from build123d import *

# Parameters (mm, degrees)
BOSS_EXTRUDE1_DEPTH = 3.175
SKETCH2_R           = 2.25
CUT_EXTRUDE1_DEPTH  = 126.120784145
FILLET1_R           = 2.54


with BuildPart() as part:
    # Sketch1 → Boss-Extrude1 (new body)
    with BuildSketch(Plane.XY):
        with BuildLine():
            Line((0, 25.4), (0, 0))
            Line((0, 0), (114.3, 0))
            Line((114.3, 0), (114.3, 50.8))
            Line((114.3, 50.8), (25.4, 50.8))
            ThreePointArc((25.4, 50.8), (17.960512242, 32.839487758), (0, 25.4))
        make_face()
    extrude(amount=BOSS_EXTRUDE1_DEPTH)

    # Sketch2 → Cut-Extrude1 (cut, through all)
    with BuildSketch(Plane.XY.offset(3.175)):
        with BuildLine():
            Line((114.3, 50.8), (69.85, 50.8))
            ThreePointArc((69.85, 50.8), (101.175009976, 37.886844698), (114.3, 6.65))
            Line((114.3, 6.65), (114.3, 50.8))
        make_face()
        with Locations((85.725, 6.65)):
            Circle(SKETCH2_R)
        with BuildLine():
            Line((90.17, 28.843472461), (33.02, 28.843472461))
            ThreePointArc((33.02, 28.843472461), (29.845, 25.668472461), (33.02, 22.493472461))
            Line((33.02, 22.493472461), (90.17, 22.493472461))
            ThreePointArc((90.17, 22.493472461), (93.345, 25.668472461), (90.17, 28.843472461))
        make_face()
        with Locations((28.575, 6.65)):
            Circle(SKETCH2_R)
    extrude(amount=-CUT_EXTRUDE1_DEPTH, mode=Mode.SUBTRACT)

    # Fillet1
    fillet1_edges = [part.edges().sort_by_distance(p)[0] for p in [
        (114.3, 0, 1.5875),
        (0, 0, 1.5875),
        (0, 25.4, 1.5875),
        (25.4, 50.8, 1.5875),
    ]]
    fillet(fillet1_edges, radius=FILLET1_R)


solid = part.part
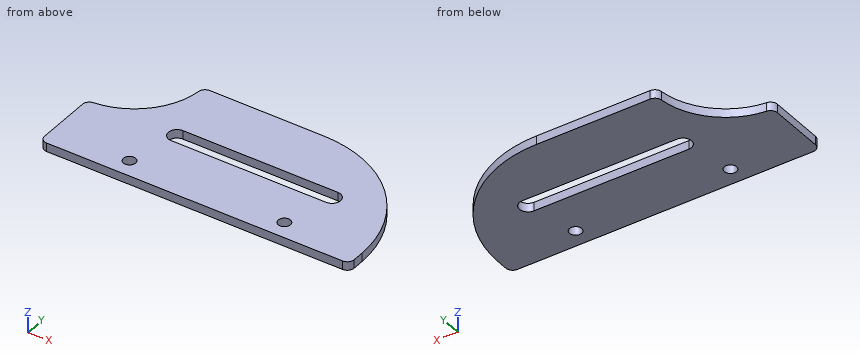
Build history of the part. All positions in model axes, mm. Round coordinates to 2 decimals unless told otherwise and drop trailing zeros. Write each loop counter-clockwise with the first axis right and the second up, starting at its lowest first coordinate (ties: lowest second). Pieces come first, ordered by that corner, then holes. Notation, with made-up numbers: (-19, -16) - (-5, -16) arc R33 cw to (-5, 13) - close; hole circle Ø10 at (70.5, 83). An arc over 180 degrees is marked (long way). Use CSV: the item, a comma, the result in double quotes.
(1) Band-saw the part on C-C (y = 27). Write the cut outline in (x, z) (3 decimals), plus the area to 3 significant figures.
Response:
outline,"(8.872, 0) - (30.138, 0) - (30.138, 3.175) - (8.872, 3.175) - close; (93.052, 0) - (109.213, 0) - (109.213, 3.175) - (93.052, 3.175) - close"
area,"119 mm²"
(2) Pin check, flat tips, straight feed: P1, Ø4, axis at x = 28.575, y = 6.65, coming from the +Z side; P2, Ø1, axis at y = 23, z = 2.5, coming from the +X side; P3, Ø6, axis at x = 24, y = 7.5, coming from the -Z side; P4, Ø1, axis at y = 43.5, z = 0.5, coming from the +X side. Stop position of each tip, or through.
Response:
P1,"through"
P2,"x = 111.26"
P3,"z = 0"
P4,"x = 95"
(3) Wall check: line 1 (Y direction, x = 61, z = 2.7); line 2 (X direction, y = 7, z = 1.75); line 3 (Y direction, x = 92.5, z = 1.45). Give the ranges that are in metal, low to high.
Response:
line 1,"0 to 22.49, 28.84 to 50.8"
line 2,"0 to 26.35, 30.8 to 83.5, 87.95 to 114.3"
line 3,"0 to 23.51, 27.83 to 44.6"
(4) Band-saw the part on B-B (z = 1.7). Write the cut outline in (x, y) (3 decimals).
Response:
outline,"(0, 2.54) arc R2.54 ccw to (2.54, 0) - (111.76, 0) arc R2.54 ccw to (114.3, 2.54) - (114.3, 6.65) arc R44.451 ccw to (69.85, 50.8) - (27.824, 50.8) arc R2.54 ccw to (25.295, 48.491) arc R25.4 cw to (2.309, 25.505) arc R2.54 ccw to (0, 22.976) - close; hole circle Ø4.5 at (28.575, 6.65); hole (33.02, 22.493) - (90.17, 22.493) arc R3.175 ccw to (90.17, 28.843) - (33.02, 28.843) arc R3.175 ccw to start; hole circle Ø4.5 at (85.725, 6.65)"
(5) Band-saw the part on A-A (x = 42). Write the cut outline in (y, z) (3 decimals).
Response:
outline,"(0, 0) - (22.493, 0) - (22.493, 3.175) - (0, 3.175) - close; (28.843, 0) - (50.8, 0) - (50.8, 3.175) - (28.843, 3.175) - close"
(6) Band-saw the part on D-D (x = 94.5). Write the cut outline in (y, z) (3 decimals).
Response:
outline,"(0, 0) - (43.339, 0) - (43.339, 3.175) - (0, 3.175) - close"
